Build history of the part. All positions in model axes, mm. A direction names the side the tool comes from. Give positions to 0.01 mm unless a question says otherwise; leave off trailing zeros. Order: outer loops, then holes, each group sorted by start corner. A loop starts at its lowest first (then second) coordinate and runs counter-clockwise, first axis right, second up. Notation, with made-up numbers: (-15, 35) - (10, 35) arc R31 ccw to (10, 61) - close; hole circle Ø3 at (62, -38.75). An arc over 180 degrees is marked (long way). Use a Markdown table: item, result. Add a question column.
(1) Slice it at D-D (x = -50). Write the cut outline in (y, z).
(2) Slice it at B-B (y = -1.5). Write the cut outline in (x, z).
(3) Slice it at A-A (z = 33). Write the cut outline in (x, y).
(4) Slice it at C-C (x = -14.5). Write the cut outline in (y, z).
(5) Flat gauge pins, fed straight in: pin 1 (4 mm diameter, centred on x = -17.5, z = 33, fed in from -Y); pin 2 (4 mm diameter, centred on x = 22.5, z = 19, fed in from -Y); pin 3 (2 mm diameter, centred on x = -1.5, z = 27.5, fed in from -Y). Where does each tip first touch, or does it go through?
(6) Which spindle directions (+Z, -Z, +X, -X, +Y, -Y) get a long thin tool onto all of the face, cutting with end or side? Do faces 1 (the face through (-44, 13, 37.338)), 2 (the face through (-6.843, -42.925, 49.86)), 3 (the face through (6.843, 42.925, 49.86)), 4 (the face through (25.5, -35.2, 49.9)), 5 (the face through (-25.5, 35.2, 49.9)). Say none if no direction does.
(7) Wall check: line 1 (Z direction, x = 28, y = 41.5); line 2 (X direction, y = 5, z = 56); line 3 (Y direction, x = -45, z = 14.5). Give the ranges that are in metal, low to high.
from build123d import *

# Parameters (mm, degrees)
F1_DEPTH = 37.338
F3_DEPTH = 25.4


with BuildPart() as f1:
    # F0 (on Top) → F1 (new body)
    with BuildSketch(Plane.XY):
        Polygon((41.884293, -50.10855), (64.294385, -11.462672), (56.62042, 32.546718), (22.453131, 61.327137), (-22.220228, 61.411907), (-56.496495, 32.761363), (-64.337424, -11.218587), (-42.074157, -49.949235), (-0.123925, -65.308081), align=None)
    extrude(amount=F1_DEPTH)

    # F2 (on face) → F3 (join)
    with BuildSketch(Plane.XY.offset(37.338)):
        Polygon((-11.20264, 45.694511), (-40.232361, 24.389435), (-45.694511, -11.20264), (-24.389435, -40.232361), (11.20264, -45.694511), (40.232361, -24.389435), (45.694511, 11.20264), (24.389435, 40.232361), align=None)
    extrude(amount=F3_DEPTH)


solid = f1.part
Solution:
| question | item | result |
|---|---|---|
| 1 | outline | (-36.16, 0) - (38.19, 0) - (38.19, 37.34) - (-36.16, 37.34) - close |
| 2 | outline | (-62.6, 0) - (62.56, 0) - (62.56, 37.34) - (43.75, 37.34) - (43.75, 62.74) - (-44.21, 62.74) - (-44.21, 37.34) - (-62.6, 37.34) - close |
| 3 | outline | (-64.34, -11.22) - (-42.07, -49.95) - (-0.12, -65.31) - (41.88, -50.11) - (64.29, -11.46) - (56.62, 32.55) - (22.45, 61.33) - (-22.22, 61.41) - (-56.5, 32.76) - close |
| 4 | outline | (-60.04, 0) - (61.4, 0) - (61.4, 37.34) - (43.27, 37.34) - (43.27, 62.74) - (-41.75, 62.74) - (-41.75, 37.34) - (-60.04, 37.34) - close |
| 5 | pin 1 | y = -59.68 |
| 5 | pin 2 | y = -57.85 |
| 5 | pin 3 | y = -65.17 |
| 6 | face 1 | +Z |
| 6 | face 2 | +Z, -X, -Y |
| 6 | face 3 | +Z, +X, +Y |
| 6 | face 4 | +Z, +X, -Y |
| 6 | face 5 | +Z, -X, +Y |
| 7 | line 1 | 0 to 37.34 |
| 7 | line 2 | -43.21 to 44.74 |
| 7 | line 3 | -44.86 to 42.37 |
